Autodesk Fusion 360 part; units mm, degrees
sketch "Sketch1" plane through (0, 0, 0) normal (0, 0, 1) x (1, 0, 0)
  line L0 (0.0245, 49.9718) -> (160.0245, 49.9718)
  line L1 (0.0257, -60.0282) -> (160.0257, -60.0282)
  arc A0 (0.0245, 49.9718) -> (0.0257, -60.0282) centre (-0.0009, -5.0282) ccw
  arc A1 (160.0257, -60.0282) -> (160.0245, 49.9718) centre (160.0195, -5.0282) ccw
  line L2 (80.0245, 49.9718) -> (80.0245, 34.9718) construction
  line L3 (0.0245, 34.9718) -> (160.0245, 34.9718)
  line L4 (80.0257, -60.0282) -> (80.0257, -45.0282) construction
  line L5 (0.0257, -45.0282) -> (160.0257, -45.0282)
  line L6 (160.0245, 49.9718) -> (160.0245, 34.9718) construction
  line L7 (160.0257, -60.0282) -> (160.0257, -45.0282) construction
  arc A2 (0.0245, 34.9718) -> (0.0257, -45.0282) centre (-0.0009, -5.0282) ccw
  arc A3 (160.0141, -45.0282) -> (160.0152, 34.9718) centre (160.0195, -5.0282) ccw
  dimension "d3" = 160
  dimension "d5" = 110
  dimension "d6" = 160
  dimension "d7" = 110
  dimension "d8" = 15
  dimension "d9" = 160
  dimension "d10" = 15
  dimension "d11" = 160
  dimension "d12" = 15
  dimension "d13" = 15
  dimension "d14" = 80
  dimension "d15" = 80
extrude "Extrude1" add sketch "Sketch1" along normal blind 20 contours L0 L1 A0 A1 | L3 L5 A2 A3
extrude "Extrude2" cut sketch "Sketch1" along normal blind 15 contours L3 L5 A2 A3
equation "length = 160 mm"
equation "width = 110 mm"
equation "d3 = length"
equation "thickness = 15 mm"
equation "d5 = width"
equation "d6 = length"
equation "d7 = width"
equation "d8 = thickness"
equation "d9 = length"
equation "d10 = thickness"
equation "d11 = length"
equation "d12 = thickness"
equation "d13 = thickness"
equation "d14 = width - thickness * 2"
equation "d15 = width - thickness * 2"
equation "o_extrude = 20 mm"
equation "i_extrude = 15 mm"
equation "d18 = o_extrude"
equation "d20 = i_extrude"
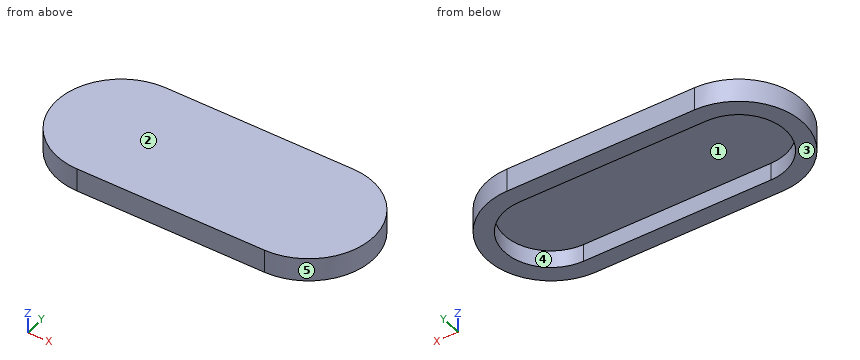
Read the model definition and answer for the solid it produces. Units are mm, in the model's axes. Face numbers are marked on the shaded views. A direction names the side the tool comes from. Give positions to 0.01 mm unless a question says otherwise; leave off trailing zeros. Write each loop counter-clockwise with the first axis right and the second up, starting at its lowest first coordinate (ties: lowest second). Pieces come first, ordered by that corner, then holes. Notation, with made-up numbers: (-16, 72) -> (26, 72) arc R14 ccw to (26, 97) -> close; hole circle Ø10 at (38, 78). An arc over 180 degrees is marked (long way). Answer as a JSON object with one key per item and string values. Group by question number.
1) Consider L1, parallel to Y at x = 70, z = 1.5; L2, parallel to X at y = -5.5, z = 5.25; L3, parallel to Z at x = 22, y = 4.5. Determine where each line is inside the solid, lowest interval first. Write a range as from..to.
2) The mould has two halves that part along Y. Classify the marked faces 3, 4 and 5: +Y half, -Y half, draft (parallel to the pull), parting line (faces both ways), or undercut.
3) Each of these flat-tipped pins is pushed along its axis until it touches: P1, Ø1, axis at x = -14, z = 16, coming from the -Y side; P2, Ø10, axis at y = 23, z = 12, coming from the -X side; P3, Ø4, axis at x = -24, z = 17, coming from the -Y side. Where does it stop, or does it pass through?
4) A tool of negligible diameter and unlimited length cuts with its end or side. For the marked faces 1 and 2, from which of +Z, -Z, +X, -X, +Y, -Y can it reach the whole face along a straight path? Write none if from no direction.
5) Find section C-C (y = 27). Write down the section's boundary in (x, z), and give its area (3 significant figures).
6) Find section A-A (z = 10.5). Write down the section's boundary in (x, y), and give its area (3 significant figures).
7) Find section B-B (x = 118). Write down the section's boundary in (y, z), and give its area (3 significant figures).
Values follow:
{
 "1": {"L1": "y = -60.03..-45.03, 34.97..49.97", "L2": "x = -55..-40, 200.02..215.02", "L3": "z = 15..20"},
 "2": {"face 3": "draft", "face 4": "undercut", "face 5": "parting line"},
 "3": {"P1": "stops at y = -58.35", "P2": "stops at x = -49.95", "P3": "stops at y = -55.44"},
 "4": {"face 1": "-Z", "face 2": "+Z, +X, -X, +Y, -Y"},
 "5": {"outline": "(-44.71, 0) -> (-23.96, 0) -> (-23.96, 15) -> (183.98, 15) -> (183.98, 0) -> (204.73, 0) -> (204.73, 20) -> (-44.71, 20) -> close", "area": "1,870 mm2"},
 "6": {"outline": "(0.02, 49.97) arc R55 ccw to (0.03, -60.03) -> (160.03, -60.03) arc R55 ccw to (160.02, 49.97) -> close; hole (0.02, 34.97) arc R40 ccw to (0.03, -45.03) -> (160.03, -45.03) arc R40 ccw to (160.02, 34.97) -> close", "area": "9,280 mm2"},
 "7": {"outline": "(-60.03, 0) -> (-45.03, 0) -> (-45.03, 15) -> (34.97, 15) -> (34.97, 0) -> (49.97, 0) -> (49.97, 20) -> (-60.03, 20) -> close", "area": "1,000 mm2"}
}
